For this review, take the finished solid that the model builds, in its own axes (mm). Coordinates: 2 decimals unless noted, no trailing zeros. Order: outer loops, then holes, each group sorted by start corner. A loop starts at its lowest first (then second) coordinate and runs counter-clockwise, first axis right, second up. Notation, with made-up numbers: (1.5, 48) -> (20.5, 48) arc R18 ccw to (20.5, 56) -> close; hole circle Ø6 at (57.5, 77.5). An arc over 180 degrees is marked (long way). Return JSON: item names as keys, results as strings. Group by question number.
Item 1: Draft analysis for pull direction X (two halves, no side actions). For faces 1 (the flat face through (40, 3.175, 0)), 2 (the cylindrical face through (-161.25, 1.57, -0.77)), 3 (the cylindrical face through (177.03, 1.57, 21.27)), state which applies: +X half, -X half, draft (parallel to the pull), parting line (faces both ways), or undercut.
Item 2: Take a section at A-A (x = -70). Write out the cut boundary in (y, z) (3 decimals), then the cut area to 3 significant figures.
Item 3: Insertion check: pin 1 (2.5 mm diameter, centred on x = 0, z = -25.4, fed in from -Y). The pin has a flat end and moves straight along its axis. Give the tip position at first contact, or say it passes through.
Item 4: Take a section at D-D (x = -122). Write out the cut boundary in (y, z) (3 decimals).
Item 5: For line 1 along Z through (x, y) = (-70, 1.6); line 2 along Z through (x, y) = (0, 1.05); line 3 along X through (y, z) = (3, 15), list the stretches that pass through material, from the lowest coordinate up.
Item 6: Take a section at C-C (z = 0). Write out the cut boundary in (x, y) (3 decimals), then the cut area to 3 significant figures.
Item 7: Take a section at B-B (y = 2.1). Count the separate pieces of the cut face and the enclosed holes in it, then the cut area to 3 significant figures.
```python
from build123d import *

# Parameters (mm, degrees)
SKETCH1_R           = 11.15
SKETCH1_R_2         = 7.5
SKETCH1_R_3         = 2.02
SKETCH1_R_4         = 3.325
BOSS_EXTRUDE1_DEPTH = 3.175


with BuildPart() as part:
    # Sketch1 → Boss-Extrude1 (new body)
    with BuildSketch(Plane(origin=(0, 0, 0), x_dir=(1, 0, 0), z_dir=(0, 1, 0))):
        with BuildLine():
            ThreePointArc((-126.258214395, 35), (-161.258214395, 0), (-126.258214395, -35))
            Line((-126.258214395, -35), (246.658214395, -35))
            Line((246.658214395, -35), (246.658214395, 35))
            Line((246.658214395, 35), (-126.258214395, 35))
        make_face()
        with Locations((-126.258214395, 0)):
            Circle(SKETCH1_R, mode=Mode.SUBTRACT)
        with Locations((-70, -17.5)):
            Circle(SKETCH1_R_2, mode=Mode.SUBTRACT)
        with Locations((0, -25.4)):
            Circle(SKETCH1_R_3, mode=Mode.SUBTRACT)
        with BuildLine():
            ThreePointArc((5, 0), (0, -5), (-5, 0))
            ThreePointArc((-5, 0), (0, 5), (5, 0))
        make_face(mode=Mode.SUBTRACT)
        with Locations((70, -17.5)):
            Circle(SKETCH1_R_2, mode=Mode.SUBTRACT)
        with Locations((173.958214395, -20)):
            Circle(SKETCH1_R_4, mode=Mode.SUBTRACT)
        with Locations((233.958214395, -20)):
            Circle(SKETCH1_R_4, mode=Mode.SUBTRACT)
        with Locations((-70, 17.5)):
            Circle(SKETCH1_R_2, mode=Mode.SUBTRACT)
        with Locations((0, 25.4)):
            Circle(SKETCH1_R_3, mode=Mode.SUBTRACT)
        with Locations((126.258214395, 0)):
            Circle(SKETCH1_R, mode=Mode.SUBTRACT)
        with Locations((70, 17.5)):
            Circle(SKETCH1_R_2, mode=Mode.SUBTRACT)
        with Locations((173.958214395, 20)):
            Circle(SKETCH1_R_4, mode=Mode.SUBTRACT)
        with Locations((233.958214395, 20)):
            Circle(SKETCH1_R_4, mode=Mode.SUBTRACT)
    extrude(amount=BOSS_EXTRUDE1_DEPTH)


solid = part.part
```
Findings below:
{
 "1": {"face 1": "draft", "face 2": "-X half", "face 3": "undercut"},
 "2": {"outline": "(0, -35) -> (3.175, -35) -> (3.175, -25) -> (0, -25) -> close; (0, -10) -> (3.175, -10) -> (3.175, 10) -> (0, 10) -> close; (0, 25) -> (3.175, 25) -> (3.175, 35) -> (0, 35) -> close", "area": "127 mm2"},
 "3": {"pin 1": "passes through"},
 "4": {"outline": "(0, -35) -> (3.175, -35) -> (3.175, -10.305) -> (0, -10.305) -> close; (0, 10.305) -> (3.175, 10.305) -> (3.175, 35) -> (0, 35) -> close"},
 "5": {"line 1": "z = -35 to -25, -10 to 10, 25 to 35", "line 2": "z = -35 to -27.42, -23.38 to -5, 5 to 23.38, 27.42 to 35", "line 3": "x = -157.88 to -77.07, -62.93 to 62.93, 77.07 to 246.66"},
 "6": {"outline": "(-161.258, 0) -> (-137.408, 0) -> (-137.408, 3.175) -> (-161.258, 3.175) -> close; (-115.108, 0) -> (-5, 0) -> (-5, 3.175) -> (-115.108, 3.175) -> close; (5, 0) -> (115.108, 0) -> (115.108, 3.175) -> (5, 3.175) -> close; (137.408, 0) -> (246.658, 0) -> (246.658, 3.175) -> (137.408, 3.175) -> close", "area": "1,120 mm2"},
 "7": {"separate pieces": "1", "enclosed holes": "13", "area": "26,300 mm2"}
}
